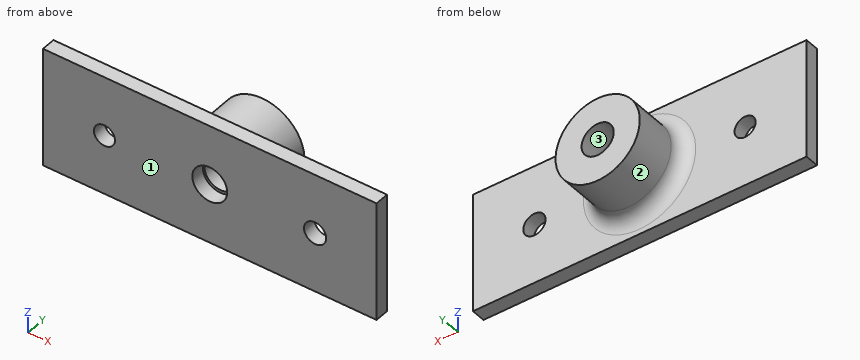
from build123d import *

# Parameters (mm, degrees)
SKETCH1_W           = 47.5
SKETCH1_H           = 17
BOSS_EXTRUDE1_DEPTH = 2
SKETCH2_R           = 2.487228871
SKETCH2_R_2         = 1.586318918
SKETCH2_R_3         = 1.5
CUT_EXTRUDE2_DEPTH  = 2
SKETCH5_R           = 6
SKETCH5_R_2         = 2.286753702
BOSS_EXTRUDE3_DEPTH = 8
FILLET1_R           = 2


with BuildPart() as part:
    # Sketch1 → Boss-Extrude1 (new body)
    with BuildSketch(Plane(origin=(0, 0, 0), x_dir=(1, 0, 0), z_dir=(0, 1, 0))):
        with Locations((-12.778061224, 6.635204082)):
            Rectangle(SKETCH1_W, SKETCH1_H)
    extrude(amount=BOSS_EXTRUDE1_DEPTH)

    # Sketch2 → Cut-Extrude2 (cut)
    with BuildSketch(Plane(origin=(0, 2, 0), x_dir=(1, 0, 0), z_dir=(0, 1, 0))):
        with Locations(Location((-12.778061224, 6.635204082, 0), (0, 0, 270))):
            Circle(SKETCH2_R)
        with Locations(Location((2.221938776, 6.635204082, 0), (0, 0, 270))):
            Circle(SKETCH2_R_2)
        with Locations(Location((-27.778061224, 6.635204082, 0), (0, 0, 270))):
            Circle(SKETCH2_R_3)
    extrude(amount=-CUT_EXTRUDE2_DEPTH, mode=Mode.SUBTRACT)

    # Sketch5 → Boss-Extrude3 (add)
    with BuildSketch(Plane(origin=(0, 2, 0), x_dir=(1, 0, 0), z_dir=(0, 1, 0))):
        with Locations(Location((-12.741585604, 6.438075133, 0), (0, 0, 270))):
            Circle(SKETCH5_R)
        with Locations(Location((-12.741585604, 6.438075133, 0), (0, 0, 280.48311938))):
            Circle(SKETCH5_R_2, mode=Mode.SUBTRACT)
    extrude(amount=BOSS_EXTRUDE3_DEPTH)

    # Fillet1
    fillet1_edges = [part.edges().sort_by_distance(p)[0] for p in [
        (-12.741585604, 2, -12.438075133),
    ]]
    fillet(fillet1_edges, radius=FILLET1_R)


solid = part.part
Build history of the part. All positions in model axes, mm. Face numbers are marked on the shaded views. Round coordinates to 2 decimals unless told otherwise and drop trailing zeros. Write each loop counter-clockwise with the first axis right and the second up, starting at its lowest first coordinate (ties: lowest second). Pieces come first, ordered by that corner, then holes. Notation, with made-up numbers: M 83,-10 L 101,-10 A6 ccw 101,-1 Z; hole C 71,25.5 d10. An arc over 180 degrees is marked long. Answer in a Markdown table with one row per item.
1. Mould opens along Z. For the marked faces 1, 2 and 3 say: +Z half, -Z half, draft (parallel to the pull), parting line (faces both ways), or undercut.
Geometry check:
| item | result |
|---|---|
| face 1 | draft |
| face 2 | parting line |
| face 3 | undercut |
2. Saw through at C-C (z = -6.5). State how many separate pieces and enclosed holes the cut face has, and give its area (3 significant figures).
Geometry check:
| item | result |
|---|---|
| separate pieces | 4 |
| enclosed holes | 0 |
| area | 134 mm2 |
3. Saw through at D-D (y = 3). List the corners of the cut face in (x, z), and give its area (3 significant figures).
Geometry check:
| item | result |
|---|---|
| outline | C -12.74,-6.44 d12.54; hole C -12.74,-6.44 d4.57 |
| area | 107 mm2 |
4. Probe L1, parallel to X at y = 1.5, z = -5.5 (3 decimals); L2, parallel to Y at x = 6, z = -7.5; L3, parallel to X at y = 4.25, z = -7. List the from-to ranges inside material, lowest first. Write a range as [from, to].
Geometry check:
| item | result |
|---|---|
| L1 | [-36.528, -28.759], [-26.798, -14.991], [-10.565, 1.114], [3.33, 10.972] |
| L2 | [0, 2] |
| L3 | [-18.72, -14.96], [-10.52, -6.77] |
5. Saw through at A-A (x = -32.5). List the corners of the cut face in (y, z), and give its area (3 significant figures).
Geometry check:
| item | result |
|---|---|
| outline | M 0,-15.14 L 2,-15.14 L 2,1.86 L 0,1.86 Z |
| area | 34.0 mm2 |
6. Saw through at B-B (y = 8.5). List the corners of the cut face in (x, z), and give its area (3 significant figures).
Geometry check:
| item | result |
|---|---|
| outline | C -12.74,-6.44 d12; hole C -12.74,-6.44 d4.57 |
| area | 96.7 mm2 |
7. Flat gauge pins, fed straight in: P1, Ø3.5, axis at x = 2.22, z = -6.64, coming from the +Y side; P2, Ø6, axis at y = 6, z = -1.5, coming from the -X side; P3, Ø6, axis at y = 8, z = -12.5, coming from the -X side; P4, Ø3, axis at x = -12.78, z = -6.64, coming from the +Y side. Where does each tip first touch, or does it go through?
Geometry check:
| item | result |
|---|---|
| P1 | y = 2 |
| P2 | x = -18.42 |
| P3 | x = -17.9 |
| P4 | through |
